from build123d import *

# Parameters (mm, degrees)
F0_R          = 15.24
F1_DEPTH      = 3.175
F2_R          = 1.651
F3_DEPTH      = 14.732
F3_DEPTH_BACK = 14.732
F4_R          = 1.5875
F5_DEPTH      = 17.145
F6_R          = 13.462
F7_DEPTH      = 6.3510001
F8_R          = 1.27


with BuildPart() as f1:
    # F0 (on Top) → F1 (new body, symmetric)
    with BuildSketch(Plane.XY):
        Circle(F0_R)
    extrude(amount=F1_DEPTH, both=True)

    # F2 (on Right) → F3 (cut, two sides)
    with BuildSketch(Plane.YZ) as f3_sk:
        Circle(F2_R)
    extrude(amount=-F3_DEPTH, mode=Mode.SUBTRACT)
    extrude(f3_sk.sketch, amount=F3_DEPTH_BACK, mode=Mode.SUBTRACT)

    # F4 (on Front) → F5 (join, symmetric)
    with BuildSketch(Plane.XZ):
        Circle(F4_R)
    extrude(amount=F5_DEPTH, both=True)

    # F6 (on face) → F7 (cut, through all)
    with BuildSketch(Plane.XY.offset(3.175)):
        Circle(F6_R)
    extrude(amount=-F7_DEPTH, mode=Mode.SUBTRACT)

    # F8
    f8_edges = [f1.edges().sort_by_distance(p)[0] for p in [
        (-1.5875, -17.145, 0),
        (-1.5875, 17.145, 0),
    ]]
    fillet(f8_edges, radius=F8_R)


solid = f1.part
Design review of the part built by this model. Coordinates are the model's own, in mm. A direction names the side the tool comes from. Coordinates: 2 decimals unless noted, no trailing zeros. Order: outer loops, then holes, each group sorted by start corner. A loop starts at its lowest first (then second) coordinate and runs counter-clockwise, first axis right, second up.
Item 1: The part is to be moulded in two halves that separate along X. For faces 4 (the cylindrical face through (12.84, 4.04, 0.04)), 5 (the flat face through (7.8, -11.2, -3.175)), 6 (the cylindrical face through (14.04, -1.65, 0.07)), 7 (the cylindrical face through (-0.34, 15.51, -1.55)), say which applies: pulls with the +X half, pulls with the -X half, needs draft (parallel to the pull), parting line crosses it, or undercut.
Item 2: Take a section at D-D, the plane x = 4.5. Write out the cut boundary in (y, z) (3 decimals).
Item 3: Take a section at A-A, the plane y = 0. Write out the cut boundary in (x, z) (3 decimals), then the cut area to 3 significant figures.
Item 4: Take a section at C-C, the plane z = -2.5. Write out the cut boundary in (x, y).
Item 5: For faces 1 (the flat face through (7.8, -11.2, 3.175)), 2 (the flat face through (-14.732, 0, 0)), 3 (the cylindrical face through (-1.586, -15.52, 0.07)), list the 3-axis set-ups (+Z, -Z, +X, -X, +Y, -Y) from which the entire face can be reached by the end or side of a thin tool; tool diameter is ignored.
Item 6: For line 1 (Y direction, x = -3, z = 0.25); line 2 (Z direction, x = 13.7, y = 0) (3 decimals); line 3 (X direction, y = -7, z = 0.25), list the stretches that pass through material, from the lowest coordinate up.
Item 7: Take a section at B-B, the plane x = -8. Write out the cut boundary in (y, z) (3 decimals).
Item 8: For pin 1 Ø2 at (y, z) = (12.5, 1) entering from +X; pin 2 Ø1 at (x, z) = (7.5, 2) entering from +Y; pin 3 Ø3 at (x, y) = (-12, -6) entering from -Z (3 decimals); pin 4 Ø3 at (y, z) = (3.5, 1.5) entering from -X, all flat-tipped, find the tip position at first contact; note any pin that passes through.
The answers:
1. face 4: undercut
1. face 5: needs draft
1. face 6: undercut
1. face 7: parting line crosses it
2. outline: (-14.56, -3.175) - (-12.688, -3.175) - (-12.688, 3.175) - (-14.56, 3.175) - close; (12.688, -3.175) - (14.56, -3.175) - (14.56, 3.175) - (12.688, 3.175) - close
3. outline: (-15.24, -3.175) - (-13.462, -3.175) - (-13.462, -1.651) - (-14.732, -1.651) - (-14.732, 1.651) - (-13.462, 1.651) - (-13.462, 3.175) - (-15.24, 3.175) - close; (13.462, -3.175) - (15.24, -3.175) - (15.24, 3.175) - (13.462, 3.175) - (13.462, 1.651) - (14.732, 1.651) - (14.732, -1.651) - (13.462, -1.651) - close
3. area: 14.2 mm2
4. outline: circle Ø30.48 at (0, 0); hole circle Ø26.92 at (0, 0)
5. face 1: +Z, +X, -X, +Y, -Y
5. face 2: none
5. face 3: -Y
6. line 1: y = -14.94 to -13.12, 13.12 to 14.94
6. line 2: z = -3.175 to -1.651, 1.651 to 3.175
6. line 3: x = -13.54 to -11.5, 11.5 to 13.54
7. outline: (-12.971, -3.175) - (-10.827, -3.175) - (-10.827, 3.175) - (-12.971, 3.175) - close; (10.827, -3.175) - (12.971, -3.175) - (12.971, 3.175) - (10.827, 3.175) - close
8. pin 1: stops at x = 10
8. pin 2: stops at y = 13.54
8. pin 3: stops at z = -3.175
8. pin 4: stops at x = -15.11
